Verification items for this drawing (mm, ordinates from the low corner). Give positions to 0.01 mm unless a question says otherwise; leave off trailing zeros. Order: outer loops, then holes, each group sorted by start corner. A loop starts at its lowest first (then second) coordinate and runs counter-clockwise, first axis right, second up.
(1) Gauge pin test, flat ends, axial feed: pin 1 (3 mm diameter, centred on x = 96.5, z = 2.5, fed in from -Y); pin 2 (1.6 mm diameter, centred on y = 57.5, z = 4, fed in from +X); pin 3 (3 mm diameter, centred on x = 98, z = 2, fed in from +Y). Record the tip position at first contact, or that the pin passes through.
(2) Sectioned sample at A-A on y = 30.5. Record the cut outline in (x, z).
(3) Sectioned sample at B-B on z = 1.85. Count the separate pieces of the cut face and the enclosed holes in it, plus the area to 3 significant figures.
(4) Sectioned sample at C-C on y = 20.5. Record the cut outline in (x, z).
(5) Scan lines: L1, parallel to X at y = 30.5, z = 4; L2, parallel to X at y = 3.5, z = 2.35; L3, parallel to Y at x = 91, z = 4.95. Record each from-to range of solid material in increasing order.
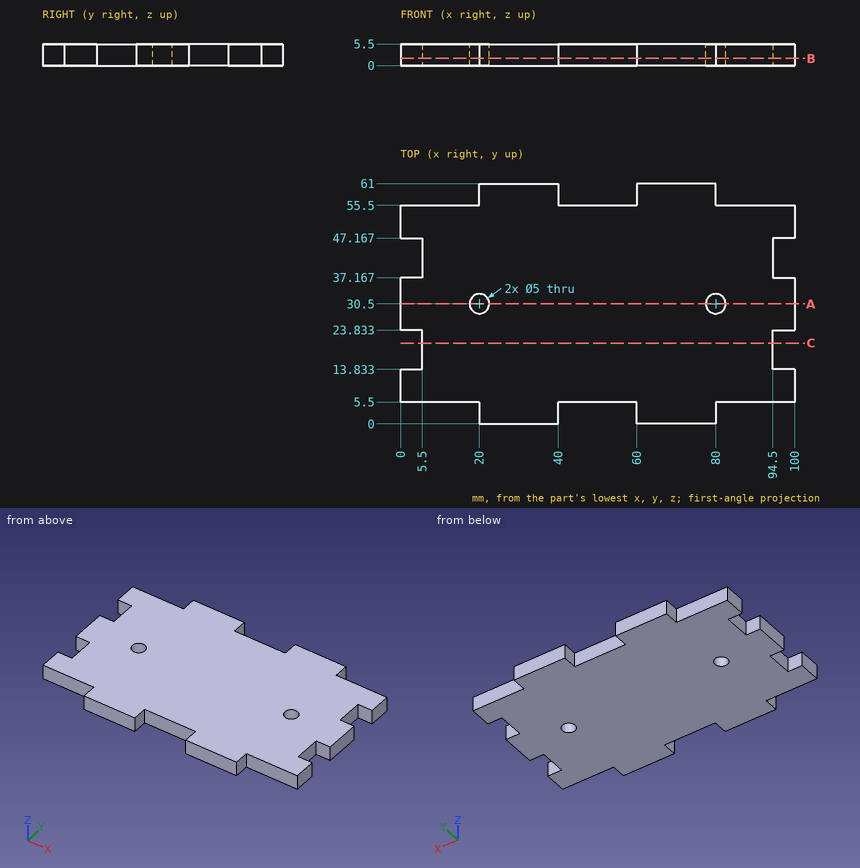
Ans:
1. pin 1: stops at y = 5.5
1. pin 2: stops at x = 80
1. pin 3: stops at y = 55.5
2. outline: (0, 0) - (17.5, 0) - (17.5, 5.5) - (0, 5.5) - close; (22.5, 0) - (77.5, 0) - (77.5, 5.5) - (22.5, 5.5) - close; (82.5, 0) - (100, 0) - (100, 5.5) - (82.5, 5.5) - close
3. separate pieces: 1
3. enclosed holes: 2
3. area: 5,180 mm2
4. outline: (5.5, 0) - (94.5, 0) - (94.5, 5.5) - (5.5, 5.5) - close
5. L1: x = 0 to 17.5, 22.5 to 77.5, 82.5 to 100
5. L2: x = 20 to 40, 60 to 80
5. L3: y = 5.5 to 55.5
